```python
from build123d import *

# Parameters (mm, degrees)
F0_R     = 5
F1_DEPTH = 25
F2_R     = 2
F3_DEPTH = 10
F5_DEPTH = 10
F7_D     = 1.2


with BuildPart() as f1:
    # F0 (on Top) → F1 (new body)
    with BuildSketch(Plane.XY):
        Circle(F0_R)
    extrude(amount=F1_DEPTH)

    # F2 (on face) → F3 (cut)
    with BuildSketch(Plane(origin=(0, 0, 0), x_dir=(1, 0, 0), z_dir=(0, 0, -1))):
        Circle(F2_R)
    extrude(amount=-F3_DEPTH, mode=Mode.SUBTRACT)

    # F4 (on face) → F5 (join)
    with BuildSketch(Plane.XY.offset(25)):
        with BuildLine():
            ThreePointArc((2, 4.582575695), (1.0215482184, 4.8945315647), (0, 5))
            ThreePointArc((0, 5), (-1.0216339401, 4.8945136727), (-2.0001605153, 4.582505637))
            Line((-2.0001605153, 4.582505637), (-2.0001605153, -4.582505637))
            ThreePointArc((-2.0001605153, -4.582505637), (-1.0216339401, -4.8945136727), (0, -5))
            ThreePointArc((0, -5), (1.0215482184, -4.8945315647), (2, -4.582575695))
            Line((2, -4.582575695), (2, 4.582575695))
        make_face()
    extrude(amount=F5_DEPTH)

    # F7 (through all)
    with Locations(Plane(origin=(-2.0001605153, 0, 0), x_dir=(0, -1, 0), z_dir=(-1, 0, 0))):
        with Locations((0, 30)):
            Hole(F7_D / 2)


solid = f1.part
```
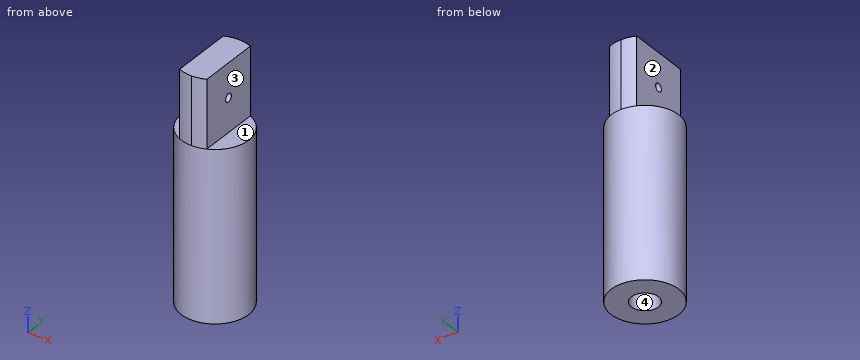
The model under review builds one solid part; all positions refer to its coordinate system, in mm. Face numbers are marked on the shaded views. Coordinates: 2 decimals unless noted, no trailing zeros. Write each loop counter-clockwise with the first axis right and the second up, starting at its lowest first coordinate (ties: lowest second). Pieces come first, ordered by that corner, then holes. Notation, with made-up numbers: (-38.5, 22) - (0.5, 22) arc R21 ccw to (0.5, 39) - close; hole circle Ø9 at (6.5, 47). An arc over 180 degrees is marked (long way). Answer in a Markdown table with one row per item. Add a question column.
Q1. Consider section A-A on z = 30. Give the boundary of the cut face in (x, y).
Q2. Consider section B-B on y = 0. Give the boundary of the cut face in (x, z).
Q3. Consider section D-D on x = -3. Give the boundary of the cut face in (y, z), then the cut area to 3 significant figures.
Q4. Clearance check with flat-ended pins moving along their axes: pin 1 (3 mm diameter, centred on x = 0.5, y = 0.5, fed in from -Z); pin 2 (1.4 mm diameter, centred on y = 0, z = 30, fed in from +X); pin 3 (5 mm diameter, centred on x = 3.5, z = 7, fed in from -Y); pin 4 (1.5 mm diameter, centred on x = 2, z = 6, fed in from -Y). State where each tip first meets the part, or that it passes through.
Q5. Consider section C-C on y = -3.75. Give the boundary of the cut face in (x, z), then the cut area to 3 significant figures.
Q6. Draft analysis for pull direction X (two halves, no side actions). For the marked faces 1, 2, 3 and 4, state which applies: +X half, -X half, draft (parallel to the pull), parting line (faces both ways), or undercut.
Q7. To check wall thickness, follow line 1 along Z through (x, y) = (0.2, 0); line 2 along Y through (x, z) = (0, 4.5); line 3 along X through (y, z) = (2, 18.5). State the ranges of each line that lie inside material, in increasing order. Write a range as from..to.
Answers below:
| question | item | result |
|---|---|---|
| 1 | outline | (-2, -4.58) arc R5 ccw to (2, -4.58) - (2, -0.6) - (-2, -0.6) - close; (-2, 0.6) - (2, 0.6) - (2, 4.58) arc R5 ccw to (-2, 4.58) - close |
| 2 | outline | (-5, 0) - (-2, 0) - (-2, 10) - (2, 10) - (2, 0) - (5, 0) - (5, 25) - (2, 25) - (2, 29.4) - (-2, 29.4) - (-2, 25) - (-5, 25) - close; (-2, 30.6) - (2, 30.6) - (2, 35) - (-2, 35) - close |
| 3 | outline | (-4, 0) - (4, 0) - (4, 25) - (-4, 25) - close |
| 3 | area | 200 mm² |
| 4 | pin 1 | z = 0 |
| 4 | pin 2 | x = 2 |
| 4 | pin 3 | y = -4.9 |
| 4 | pin 4 | y = -4.84 |
| 5 | outline | (-3.31, 0) - (3.31, 0) - (3.31, 25) - (2, 25) - (2, 35) - (-2, 35) - (-2, 25) - (-3.31, 25) - close |
| 5 | area | 205 mm² |
| 6 | face 1 | draft |
| 6 | face 2 | -X half |
| 6 | face 3 | +X half |
| 6 | face 4 | undercut |
| 7 | line 1 | 10..29.4, 30.6..35 |
| 7 | line 2 | -5..-2, 2..5 |
| 7 | line 3 | -4.58..4.58 |
